Check sheet for the drawn part. Datum: minimum x, y, z corner. Units: mm. A direction names the side the tool comes from. Round coordinates to 2 decimals unless told otherwise and drop trailing zeros. Write each loop counter-clockwise with the first axis right and the second up, starting at its lowest first coordinate (ties: lowest second). Pieces come first, ordered by that corner, then holes. Notation, with made-up numbers: (-38.75, 47.25) - (-10.75, 47.25) arc R25 ccw to (-10.75, 67.25) - close; hole circle Ø8 at (66, -16.5). An arc over 180 degrees is marked (long way). Write each question's results on one line, items separated by ' | '.
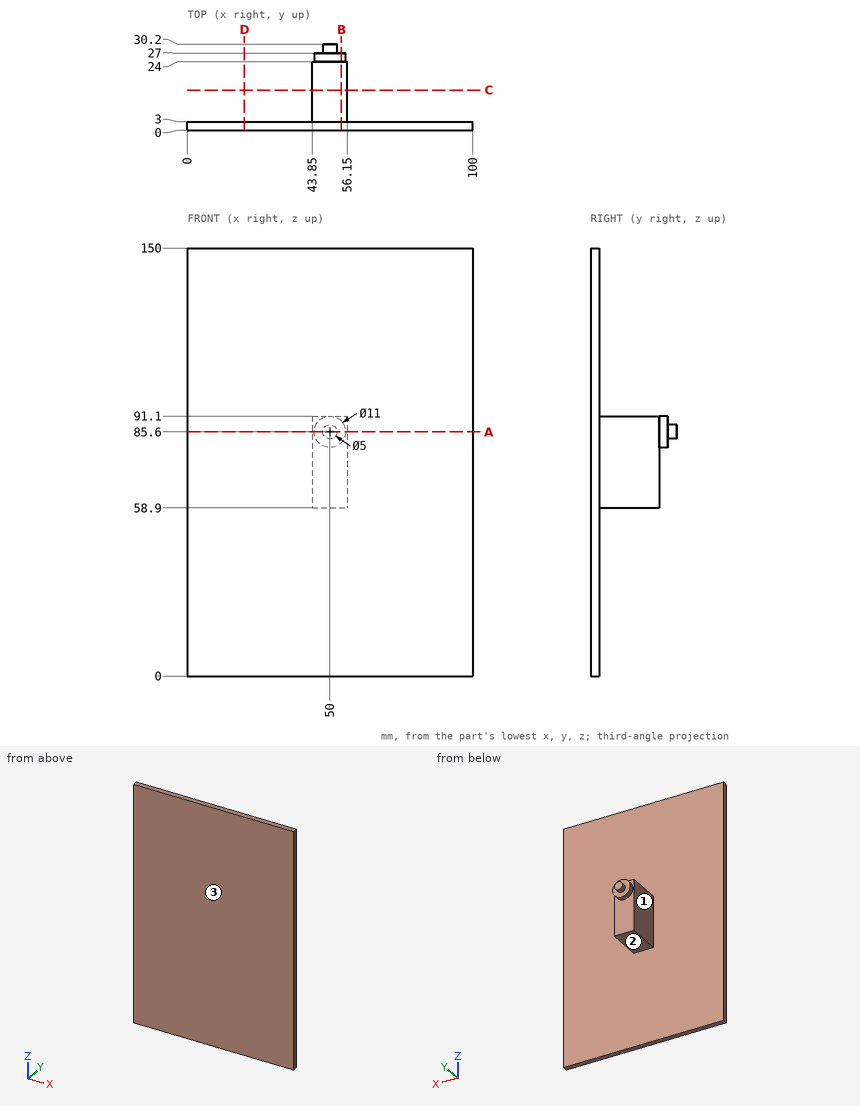
(1) Section check A-A (z = 85.6). Record the cut outline in (x, y).
Answer:
outline: (0, 0) - (100, 0) - (100, 3) - (56.15, 3) - (56.15, 24) - (55.5, 24) - (55.5, 27) - (52.5, 27) - (52.5, 30.2) - (47.5, 30.2) - (47.5, 27) - (44.5, 27) - (44.5, 24) - (43.85, 24) - (43.85, 3) - (0, 3) - close
(2) Thickness scan on L1, parallel to Y at x = 88, z = 33; L2, parallel to Z at x = 53.5, y = 21; L3, parallel to X at y = 16, z = 74. Record the ranges inside material, lowest first.
Answer:
L1: 0 to 3 | L2: 58.9 to 91.1 | L3: 43.85 to 56.15
(3) Section check B-B (x = 54). Record the cut outline in (y, z).
Answer:
outline: (0, 0) - (3, 0) - (3, 58.9) - (24, 58.9) - (24, 81.83) - (27, 81.83) - (27, 89.37) - (24, 89.37) - (24, 91.1) - (3, 91.1) - (3, 150) - (0, 150) - close
(4) Section check D-D (x = 20). Record the cut outline in (y, z).
Answer:
outline: (0, 0) - (3, 0) - (3, 150) - (0, 150) - close
(5) Go/stop test with flat-tipped pins: pin 1 Ø10 at (x, y) = (50, 18.5) entering from -Z; pin 2 Ø6 at (x, z) = (49, 69.5) entering from +Y; pin 3 Ø17 at (y, z) = (14, 69.5) entering from +X. Record where each tip stops, or that it passes through.
Answer:
pin 1: z = 58.9 | pin 2: y = 24 | pin 3: x = 56.15
(6) Set-up check for the marked faces 1, 2 and 3: record each of +Z, -Z, +X, -X, +Y, -Y from which the full face is reachable in a straight line by a thin tool's end or side.
Answer:
face 1: +Z, -Z, -X, +Y | face 2: -Z, +X, -X, +Y | face 3: +Z, -Z, +X, -X, -Y
(7) Section check C-C (y = 14). Record the cut outline in (x, z).
Answer:
outline: (43.85, 58.9) - (56.15, 58.9) - (56.15, 91.1) - (43.85, 91.1) - close
